from build123d import *

# Parameters (mm, degrees)
SKETCH1_R               = 55
SKETCH1_R_2             = 4
BOSS_EXTRUDE1_DEPTH     = 21
SKETCH2_R               = 3
CUT_EXTRUDE3_DEPTH      = 22
CUT_EXTRUDE3_DEPTH_BACK = 10
SKETCH3_R               = 5
CUT_EXTRUDE4_DEPTH      = 6


with BuildPart() as part:
    # Sketch1 → Boss-Extrude1 (new body)
    with BuildSketch(Plane(origin=(0, 0, 0), x_dir=(1, 0, 0), z_dir=(0, 1, 0))):
        Circle(SKETCH1_R)
        Circle(SKETCH1_R_2, mode=Mode.SUBTRACT)
    extrude(amount=BOSS_EXTRUDE1_DEPTH)

    # Sketch2 → Cut-Extrude3 (cut, two sides)
    with BuildSketch(Plane(origin=(0, 0, 0), x_dir=(1, 0, 0), z_dir=(0, 1, 0))) as cut_extrude3_sk:
        with Locations((37.5, 20)):
            Circle(SKETCH2_R)
        with Locations((37.5, -20)):
            Circle(SKETCH2_R)
        with Locations((-37.5, -20)):
            Circle(SKETCH2_R)
        with Locations((-37.5, 20)):
            Circle(SKETCH2_R)
        with Locations((0, 42.5)):
            Circle(SKETCH2_R)
        with Locations((0, -42.5)):
            Circle(SKETCH2_R)
    extrude(amount=CUT_EXTRUDE3_DEPTH, mode=Mode.SUBTRACT)
    extrude(cut_extrude3_sk.sketch, amount=-CUT_EXTRUDE3_DEPTH_BACK, mode=Mode.SUBTRACT)

    # Sketch3 → Cut-Extrude4 (cut)
    with BuildSketch(Plane(origin=(0, 0, 0), x_dir=(1, 0, 0), z_dir=(0, 1, 0))):
        with Locations((-37.5, 20)):
            Circle(SKETCH3_R)
        with Locations((-37.5, -20)):
            Circle(SKETCH3_R)
        with Locations((37.5, 20)):
            Circle(SKETCH3_R)
        with Locations((37.5, -20)):
            Circle(SKETCH3_R)
        with Locations((0, 42.5)):
            Circle(SKETCH3_R)
        with Locations((0, -42.5)):
            Circle(SKETCH3_R)
    extrude(amount=CUT_EXTRUDE4_DEPTH, mode=Mode.SUBTRACT)


solid = part.part
CAD build for the part. Positions are in the model's coordinates, mm. A direction names the side the tool comes from. Round coordinates to 2 decimals unless told otherwise and drop trailing zeros. Order: outer loops, then holes, each group sorted by start corner. A loop starts at its lowest first (then second) coordinate and runs counter-clockwise, first axis right, second up. Notation, with made-up numbers: (22.25, 3) -> (31.25, 3) arc R17 cw to (31.25, 25) -> close; hole circle Ø3 at (59.5, 75). An arc over 180 degrees is marked (long way). Write item = value, one per line. Start each with the question number.
(1) Probe line 1 (Z direction, x = 37.5, y = 3.85); line 2 (Z direction, x = -37.5, y = 17); line 3 (X direction, y = 14, z = 0). List the from-to ranges inside material, lowest first. Write a range as [from, to].
(2) Pin check, flat tips, straight feed: P1, Ø3, axis at x = 2, z = 44, coming from the -Y side; P2, Ø1, axis at y = 9.5, z = 37, coming from the -X side; P3, Ø4, axis at x = -11.5, y = 5, coming from the -Z side. Stop position of each tip, or through.
(3) Cut at D-D, the plane x = -37.5. List the corners of the cut face in (y, z), then the cut area to 3 significant figures.
(4) Which spindle directions (+Z, -Z, +X, -X, +Y, -Y) get a long thin tool onto all of the face, cutting with end or side? Do faces 1 (the cylindrical face through (-40.5, 13.4, -20.1)), 2 (the flat face through (-35, 6, 22)). Say none if no direction does.
(5) Cut at B-B, the plane x = 0. List the corners of the cut face in (y, z), then the cut area to 3 significant figures.
(6) Cut at C-C, the plane z = 0. List the corners of the cut face in (x, y), then the cut area to 3 significant figures.
(7) Pull direction Z, two halves, no side cores. Call faces 3 (the cylindrical face through (34.5, 13.4, 19.9)), 4 (the cylindrical face through (-11.923, 10.353, 53.692)), 5 (the flat face through (40, 6, -18)), 6 (the flat face through (11, 0, -1)): released by +Z, released by -Z, zero draft, split by the parting line, or undercut.
(8) Cut at A-A, the plane y = 14.5. List the corners of the cut face in (x, z).
Model answer:
q1.line_1 = [-40.23, -25], [-15, 15], [25, 40.23]
q1.line_2 = [-40.23, -23], [-17, 17], [23, 40.23]
q1.line_3 = [-55, -4], [4, 55]
q2.P1 = 6
q2.P2 = -41.14
q2.P3 = -54.17
q3.outline = (0, -40.23) -> (21, -40.23) -> (21, -23) -> (6, -23) -> (6, -25) -> (0, -25) -> close; (0, -15) -> (6, -15) -> (6, -17) -> (21, -17) -> (21, 17) -> (6, 17) -> (6, 15) -> (0, 15) -> close; (0, 25) -> (6, 25) -> (6, 23) -> (21, 23) -> (21, 40.23) -> (0, 40.23) -> close
q3.area = 1,390 mm2
q4.face_1 = +Y, -Y
q4.face_2 = -Y
q5.outline = (0, -55) -> (21, -55) -> (21, -45.5) -> (6, -45.5) -> (6, -47.5) -> (0, -47.5) -> close; (0, -37.5) -> (6, -37.5) -> (6, -39.5) -> (21, -39.5) -> (21, -4) -> (0, -4) -> close; (0, 4) -> (21, 4) -> (21, 39.5) -> (6, 39.5) -> (6, 37.5) -> (0, 37.5) -> close; (0, 47.5) -> (6, 47.5) -> (6, 45.5) -> (21, 45.5) -> (21, 55) -> (0, 55) -> close
q5.area = 1,840 mm2
q6.outline = (-55, 0) -> (-4, 0) -> (-4, 21) -> (-55, 21) -> close; (4, 0) -> (55, 0) -> (55, 21) -> (4, 21) -> close
q6.area = 2,140 mm2
q7.face_3 = undercut
q7.face_4 = split by the parting line
q7.face_5 = undercut
q7.face_6 = zero draft
q8.outline = circle Ø110 at (0, 0); hole circle Ø6 at (-37.5, -20); hole circle Ø6 at (-37.5, 20); hole circle Ø8 at (0, 0); hole circle Ø6 at (0, -42.5); hole circle Ø6 at (0, 42.5); hole circle Ø6 at (37.5, -20); hole circle Ø6 at (37.5, 20)
